Read the model definition and answer for the solid it produces. Units are mm, in the model's axes. A direction names the side the tool comes from. Coordinates: 2 decimals unless noted, no trailing zeros. Write each loop counter-clockwise with the first axis right and the second up, starting at its lowest first coordinate (ties: lowest second). Pieces come first, ordered by that corner, then holes. Notation, with made-up numbers: M -28.5,37.25 L -11.5,37.25 A8 ccw -11.5,41.25 Z; hole C -28,-1 d10. An arc over 180 degrees is marked long. Write item = value, one per line.
from build123d import *

# Parameters (mm, degrees)
SKETCH1_W                                            = 60
SKETCH1_H                                            = 60
BOSS_EXTRUDE1_DEPTH                                  = 5
CSK_FOR_M5_HEX_SOCKET_COUNTERSUNK_CAP_SC_D           = 5.8
CSK_FOR_M5_HEX_SOCKET_COUNTERSUNK_CAP_SC_DEPTH       = 5
CSK_FOR_M5_HEX_SOCKET_COUNTERSUNK_CAP_SC_CSINK_D     = 11.2
CSK_FOR_M5_HEX_SOCKET_COUNTERSUNK_CAP_SC_CSINK_ANGLE = 90
CSK_FOR_M5_HEX_SOCKET_COUNTERSUNK_CAP_SC_TIP         = 1.742495795
BOSS_EXTRUDE2_DEPTH                                  = 30
FILLET1_R                                            = 10
CUT_EXTRUDE1_REACH                                   = 73.553
SKETCH11_R                                           = 4.15
CIRPATTERN1_COUNT                                    = 4
FILLET2_R                                            = 10
CUT_EXTRUDE2_DEPTH                                   = 6.5
CIRPATTERN2_COUNT                                    = 4


with BuildPart() as part:
    # Sketch1 → Boss-Extrude1 (new body)
    with BuildSketch(Plane.XY):
        with Locations((-22.5, 22.5)):
            Rectangle(SKETCH1_W, SKETCH1_H)
    extrude(amount=BOSS_EXTRUDE1_DEPTH)

    # CSK for M5 Hex Socket Countersunk Cap Screw1
    with Locations(Plane(origin=(0, 0, 0), x_dir=(-1, 0, 0), z_dir=(0, 0, -1))):
        with Locations((2.5, 42.5), (42.5, 42.5), (42.5, 2.5), (2.5, 2.5)):
            CounterSinkHole(CSK_FOR_M5_HEX_SOCKET_COUNTERSUNK_CAP_SC_D / 2, CSK_FOR_M5_HEX_SOCKET_COUNTERSUNK_CAP_SC_CSINK_D / 2, depth=CSK_FOR_M5_HEX_SOCKET_COUNTERSUNK_CAP_SC_DEPTH, counter_sink_angle=CSK_FOR_M5_HEX_SOCKET_COUNTERSUNK_CAP_SC_CSINK_ANGLE)
            with Locations((0, 0, -(CSK_FOR_M5_HEX_SOCKET_COUNTERSUNK_CAP_SC_DEPTH + CSK_FOR_M5_HEX_SOCKET_COUNTERSUNK_CAP_SC_TIP / 2))):  # 118° drill point
                Cone(0, CSK_FOR_M5_HEX_SOCKET_COUNTERSUNK_CAP_SC_D / 2, CSK_FOR_M5_HEX_SOCKET_COUNTERSUNK_CAP_SC_TIP, mode=Mode.SUBTRACT)

    # Sketch8 → Boss-Extrude2 (add)
    with BuildSketch(Plane(origin=(0, 0, 0), x_dir=(-1, 0, 0), z_dir=(0, 0, -1))):
        Polygon((27, 0), (27, 6.5), (31.5, 6.5), (31.5, 10), (27.257359313, 14.242640687), (17.742640687, 14.242640687), (13.5, 10), (13.5, 6.5), (18, 6.5), (18, 0), align=None)
        Polygon((0, 18), (6.5, 18), (6.5, 13.5), (10, 13.5), (14.242640687, 17.742640687), (14.242640687, 27.257359313), (10, 31.5), (6.5, 31.5), (6.5, 27), (0, 27), align=None)
        Polygon((18, 45), (18, 38.5), (13.5, 38.5), (13.5, 35), (17.742640687, 30.757359313), (27.257359313, 30.757359313), (31.5, 35), (31.5, 38.5), (27, 38.5), (27, 45), align=None)
        Polygon((45, 27), (38.5, 27), (38.5, 31.5), (35, 31.5), (30.757359313, 27.257359313), (30.757359313, 17.742640687), (35, 13.5), (38.5, 13.5), (38.5, 18), (45, 18), align=None)
    extrude(amount=BOSS_EXTRUDE2_DEPTH)

    # Fillet1
    # the kernel refuses this fillet: 10 mm, written as the material it adds along each edge
    with BuildSketch(Plane(origin=(-27, 45, 0), x_dir=(0, 1, 0), z_dir=(1, 0, 0)), Plane(origin=(-45, 18, 0), x_dir=(-1, 0, 0), z_dir=(0, 1, 0)), Plane(origin=(0, 27, 0), x_dir=(1, 0, 0), z_dir=(0, -1, 0)), Plane(origin=(-18, 0, 0), x_dir=(0, -1, 0), z_dir=(-1, 0, 0))) as fillet1_piece_1:
        with BuildLine():
            CenterArc((10, -9.682458366), FILLET1_R, 104.477512186, 75.522487814)
            Line((0, -9.682458366), (0, 0))
            Line((0, 0), (7.5, 0))
        make_face()
    extrude(amount=9)
    # the kernel refuses this fillet: 10 mm, written as the material it takes off along each edge
    with BuildSketch(Plane(origin=(-52, 45, -30), x_dir=(0, -1, 0), z_dir=(1, 0, 0)), Plane(origin=(7, 0, -30), x_dir=(0, 1, 0), z_dir=(-1, 0, 0))) as fillet1_2_piece_1:
        with BuildLine():
            CenterArc((FILLET1_R, -FILLET1_R), FILLET1_R, 90, 90)
            Line((0, -FILLET1_R), (0, 0))
            Line((0, 0), (FILLET1_R, 0))
        make_face()
    extrude(amount=59, mode=Mode.SUBTRACT)
    with BuildSketch(Plane(origin=(-45, -7, -30), x_dir=(0, 0, 1), z_dir=(0, 1, 0)), Plane(origin=(0, 52, -30), x_dir=(0, 0, 1), z_dir=(0, -1, 0))) as fillet1_2_piece_2:
        with BuildLine():
            CenterArc((FILLET1_R, FILLET1_R), FILLET1_R, 180, 90)
            Line((0, FILLET1_R), (0, 0))
            Line((0, 0), (FILLET1_R, 0))
        make_face()
    extrude(amount=59, mode=Mode.SUBTRACT)

    # Sketch11 → Cut-Extrude1 (cut, up to next)
    with BuildSketch(Plane(origin=(0, 14.242640687, 0), x_dir=(1, 0, 0), z_dir=(0, 1, 0)), mode=Mode.PRIVATE) as cut_extrude1_sk1:
        with Locations(Location((-22.5, 15, 0), (0, 0, 180))):
            Circle(SKETCH11_R)
    cut_extrude1_tool1 = extrude(cut_extrude1_sk1.sketch, amount=-CUT_EXTRUDE1_REACH, mode=Mode.PRIVATE) & part.part
    cut_extrude1 = cut_extrude1_tool1.solids().sort_by_distance((-22.5, 14.242641, -15))[0]
    add(cut_extrude1, mode=Mode.SUBTRACT)

    # CirPattern1: Cut-Extrude1 ×4 about axis
    cirpattern1_axis = Axis((-22.5, 22.5, 0), (0, 0, -1))
    for i in range(1, CIRPATTERN1_COUNT):
        add(cut_extrude1.rotate(cirpattern1_axis, i * 360 / CIRPATTERN1_COUNT), mode=Mode.SUBTRACT)

    # Fillet2
    fillet2_edges = [part.edges().sort_by_distance(p)[0] for p in [
        (7.5, 52.5, 2.5),
        (7.5, -7.5, 2.5),
        (-52.5, -7.5, 2.5),
        (-52.5, 52.5, 2.5),
    ]]
    fillet(fillet2_edges, radius=FILLET2_R)

    # Sketch12 → Cut-Extrude2 (cut)
    with BuildSketch(Plane(origin=(-30.757359313, 0, 0), x_dir=(0, 0, -1), z_dir=(1, 0, 0))):
        Polygon((11.102885683, 15.75), (18.897114317, 15.75), (22.794228634, 22.5), (18.897114317, 29.25), (11.102885683, 29.25), (7.205771366, 22.5), align=None)
    cut_extrude2 = extrude(amount=-CUT_EXTRUDE2_DEPTH, mode=Mode.SUBTRACT)

    # CirPattern2: Cut-Extrude2 ×4 about axis
    cirpattern2_axis = Axis((-22.5, 22.5, 0), (0, 0, 1))
    for i in range(1, CIRPATTERN2_COUNT):
        add(cut_extrude2.rotate(cirpattern2_axis, i * 360 / CIRPATTERN2_COUNT), mode=Mode.SUBTRACT)


solid = part.part
Item 1: Flat-ended cylindrical pins translate along their axes: pin 1 (2 mm diameter, centred on y = 16, z = -10, fed in from +X); pin 2 (12 mm diameter, centred on x = -14, z = -17, fed in from +Y); pin 3 (11 mm diameter, centred on y = -2.5, z = -12.5, fed in from +X); pin 4 (18 mm diameter, centred on x = -25, y = 30, fed in from -Z). Find the tip coordinate at first contact, or state that the pin passes through.
Worked answers:
pin_1 = -6.5
pin_2 = 45
pin_3 = -18
pin_4 = -30
Item 2: Consider line 1 along Y through (x, z) = (-42.5, 4.1); line 2 along Y through (x, z) = (-28, -3); line 3 along Z through (x, y) = (-23, 31). Determine where each line is inside the solid, lowest interval first. Write a range as from..to.
Worked answers:
line_1 = -7.5..-0.4, 5.4..39.6, 45.4..52.5
line_2 = 6.5..13.5, 31.5..38.5
line_3 = -30..-22.51, -7.49..5
Item 3: Which of the six approach directions +Z, -Z, +X, -X, +Y, -Y give full straight-line access (tool end or side, diameter ignored) to faces 4 (the face through (-42, 27, -11)), 5 (the face through (-45, 20, -11)), 6 (the face through (-37, 13.5, -15)), 7 (the face through (-7.743, 19, -18))?
Worked answers:
face_4 = -Z, -X, +Y
face_5 = -Z, -X, +Y, -Y
face_6 = -Z, -X, -Y
face_7 = none
Item 4: Find section A-A (y = 21.5). State how many separate pieces and enclosed holes the cut face has, and give its area (3 significant figures).
Worked answers:
separate_pieces = 3
enclosed_holes = 0
area = 837 mm²
Item 5: Find section D-D (y = 36). Determine the outline of the cut face in (x, z), and give its area (3 significant figures).
Worked answers:
outline = M -52.5,0 L -31.5,0 L -31.5,-29.95 L -13.5,-29.95 L -13.5,0 L 7.5,0 L 7.5,5 L -52.5,5 Z; hole M -29.25,-18.9 L -22.5,-22.79 L -15.75,-18.9 L -15.75,-11.1 L -22.5,-7.21 L -29.25,-11.1 Z
area = 681 mm²
Item 6: For a pull along Z with two mould halves and no side action, classify faces 1 (the face through (-10, 29.25, -15)), 2 (the face through (-6.5, 16, -14)), 3 (the face through (2.15, 22.56, -3.49)) as released by +Z, released by -Z, zero draft, split by the parting line, or undercut.
Worked answers:
face_1 = undercut
face_2 = zero draft
face_3 = released by -Z
